Check sheet for the drawn part. Datum: minimum x, y, z corner. Units: mm. A direction names the side the tool comes from. Coordinates: 2 decimals unless noted, no trailing zeros. Write each loop counter-clockwise with the first axis right and the second up, starting at its lowest first coordinate (ties: lowest second). Pieces come first, ordered by that corner, then holes. Notation, with made-up numbers: (76.25, 8.25) -> (120.25, 8.25) arc R22 cw to (120.25, 42.25) -> close; hole circle Ø9 at (29, -0.75). An arc over 180 degrees is marked (long way). Write item = value, one per line. Start each with the question number.
(1) Set-up check for the marked faces 5, 6 and 7: record each of +Z, -Z, +X, -X, +Y, -Y from which the full face is reachable in a straight line by a thin tool's end or side.
(2) Mould release check, pull along Y, two halves, no side actions. Record for the marked faces 1, 2, 3 and 4: released by +Y, released by -Y, zero draft, split by the parting line, or undercut.
(3) Gauge pin test, flat ends, axial feed: pin 1 Ø15 at (x, z) = (41, 11.5) entering from -Y; pin 2 Ø1 at (y, z) = (34.5, 6.5) entering from +X. Record the tip position at first contact, or that the pin passes through.
(4) Material ranges on probe 1 along Y at (x, z) = (67, 26); probe 2 along X at (y, z) = (9, 20); probe 3 along Z at (x, y) = (27, 52), recorded low to high. Write a range as [from, to].
(5) Section check A-A (y = 7.5). Record the cut outline in (x, z).
(6) Section check C-C (x = 17). Record the cut outline in (y, z).
(7) Section check D-D (y = 46.5). Record the cut outline in (x, z).
(8) Section check B-B (z = 26.5). Record the cut outline in (x, y).
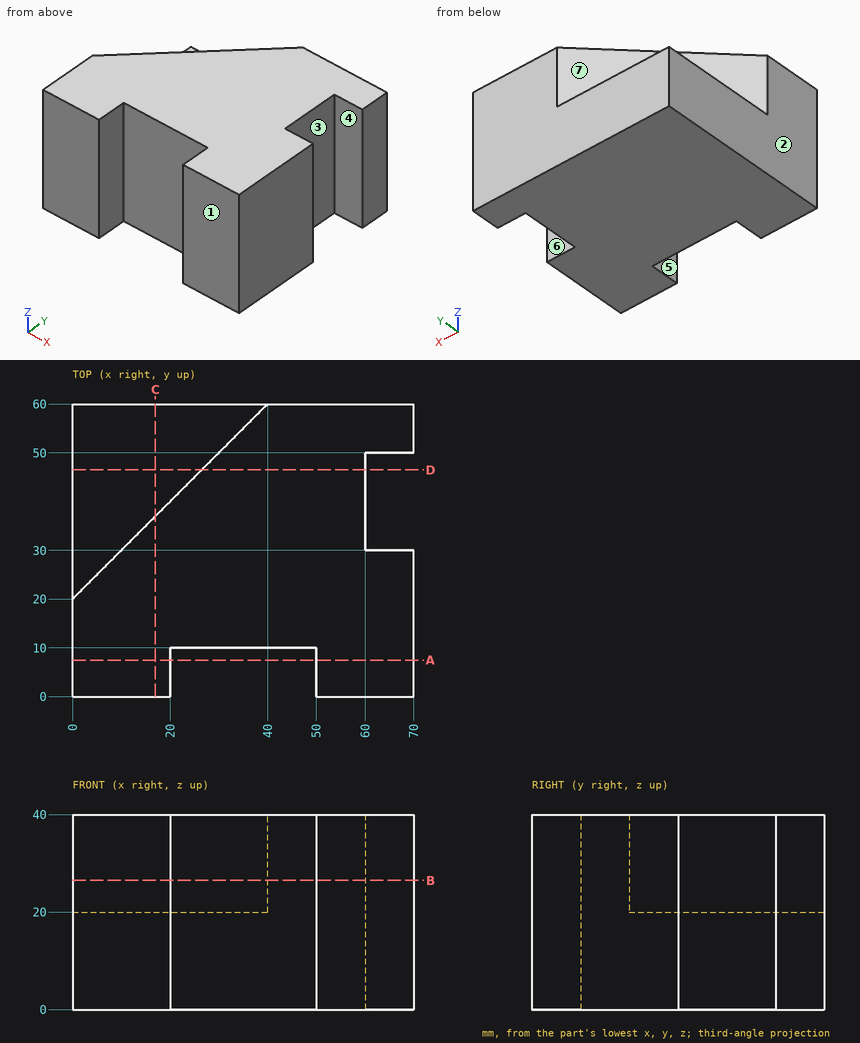
Response:
q1.face_5 = +Z, -Z, -Y
q1.face_6 = +Z, -Z, +X
q1.face_7 = +Z, -X, +Y
q2.face_1 = released by -Y
q2.face_2 = zero draft
q2.face_3 = undercut
q2.face_4 = undercut
q3.pin_1 = 10
q3.pin_2 = 60
q4.probe_1 = [0, 30], [50, 60]
q4.probe_2 = [0, 20], [50, 70]
q4.probe_3 = [0, 20]
q5.outline = (0, 0) -> (20, 0) -> (20, 40) -> (0, 40) -> close; (50, 0) -> (70, 0) -> (70, 40) -> (50, 40) -> close
q6.outline = (0, 0) -> (60, 0) -> (60, 20) -> (37, 20) -> (37, 40) -> (0, 40) -> close
q7.outline = (0, 0) -> (60, 0) -> (60, 40) -> (26.5, 40) -> (26.5, 20) -> (0, 20) -> close
q8.outline = (0, 0) -> (20, 0) -> (20, 10) -> (50, 10) -> (50, 0) -> (70, 0) -> (70, 30) -> (60, 30) -> (60, 50) -> (70, 50) -> (70, 60) -> (40, 60) -> (0, 20) -> close
